The model under review builds one solid part; all positions refer to its coordinate system, in mm. A direction names the side the tool comes from. Round coordinates to 2 decimals unless told otherwise and drop trailing zeros. Write each loop counter-clockwise with the first axis right and the second up, starting at its lowest first coordinate (ties: lowest second). Pieces come first, ordered by that corner, then holes. Notation, with made-up numbers: (35, 84) - (79, 84) arc R33 cw to (79, 123) - close; hole circle Ø10 at (0, -24.75). An arc over 180 degrees is marked (long way). Use one line per item in the form item = value.
from build123d import *

# Parameters (mm, degrees)
FEMALE_HEX_STANDOFF_SKETCH_R  = 1.51
FEMALE_HEX_STANDOFF_DEPTH     = 5
STUD_ROOT_SKETCH_R            = 1.85
STUD_ROOT_DEPTH               = 0.45
MALE_THREAD_ENVELOPE_START    = -8
MALE_THREAD_ENVELOPE_SKETCH_R = 1.5
MALE_THREAD_ENVELOPE_DEPTH    = 8


with BuildPart() as part:
    # Female_hex_standoff_Sketch → Female_hex_standoff (new body)
    with BuildSketch(Plane.XY):
        Polygon((3.175426481, 0), (1.58771324, 2.75), (-1.58771324, 2.75), (-3.175426481, 0), (-1.58771324, -2.75), (1.58771324, -2.75), align=None)
        Circle(FEMALE_HEX_STANDOFF_SKETCH_R, mode=Mode.SUBTRACT)
    extrude(amount=FEMALE_HEX_STANDOFF_DEPTH)

    # Stud_root_Sketch → Stud_root (add)
    with BuildSketch(Plane.XY):
        Circle(STUD_ROOT_SKETCH_R)
    extrude(amount=STUD_ROOT_DEPTH)

    # Male_thread_envelope_Sketch → Male_thread_envelope (add)
    with BuildSketch(Plane.XY.offset(MALE_THREAD_ENVELOPE_START)):
        Circle(MALE_THREAD_ENVELOPE_SKETCH_R)
    extrude(amount=MALE_THREAD_ENVELOPE_DEPTH)


solid = part.part
(1) The part is to be moulded in two halves that separate along X. For faces 1 (the cylindrical face through (-1.5, 0.07, -4.06)), 2 (the cylindrical face through (-0.197, 1.497, 2.693)), 3 (the flat face through (0, 2.75, 2)), say which applies: +X half, -X half, draft (parallel to the pull), parting line (faces both ways), or undercut.
Geometry results:
face_1 = parting line
face_2 = undercut
face_3 = draft
(2) Add section A-A on x = 0. Write out the cut boundary in (y, z).
Geometry results:
outline = (-2.75, 0) - (-1.5, 0) - (-1.5, -8) - (1.5, -8) - (1.5, 0) - (2.75, 0) - (2.75, 5) - (1.51, 5) - (1.51, 0.45) - (-1.51, 0.45) - (-1.51, 5) - (-2.75, 5) - close
(3) Machinability: for faces 4 (the flat face through (1.4, 1.3, 0)), 5 (the flat face through (0, 0, 0.45)), 6 (the flat face through (2.37, -1.394, 2.465)), which of the approach directions +Z, -Z, +X, -X, +Y, -Y give a long, thin tool a straight path to every point of the face, cutting with its end or side? Answer none if there is none.
Geometry results:
face_4 = -Z
face_5 = +Z
face_6 = +Z, -Z, +X, -Y
(4) Insertion check: P1, Ø1.5, axis at x = 0, y = 0.5, coming from the +Z side. The pin has a flat end and moves straight along its axis. Give the tip position at first contact, or say it passes through.
Geometry results:
P1 = 0.45
(5) Add section C-C on z = -1.75. Write out the cut boundary in (x, y).
Geometry results:
outline = circle Ø3 at (0, 0)
(6) To check wall thickness, follow L1, parallel to Y at x = 0, z = 2.45; L2, parallel to Z at x = -0.5, y = -1.9; L3, parallel to Z at x = 0.25, y = 0.2. State the ranges of each line that lie inside material, in increasing order.
Geometry results:
L1 = -2.75 to -1.51, 1.51 to 2.75
L2 = 0 to 5
L3 = -8 to 0.45
(7) Add section D-D on y = -1.7. Write out the cut boundary in (x, z), then the cut area to 3 significant figures.
Geometry results:
outline = (-2.19, 0) - (2.19, 0) - (2.19, 5) - (-2.19, 5) - close
area = 21.9 mm2
(8) Add section B-B on y = 0.4. Write out the cut boundary in (x, z), then the cut area to 3 significant figures.
Geometry results:
outline = (-2.94, 0) - (-1.45, 0) - (-1.45, -8) - (1.45, -8) - (1.45, 0) - (2.94, 0) - (2.94, 5) - (1.46, 5) - (1.46, 0.45) - (-1.46, 0.45) - (-1.46, 5) - (-2.94, 5) - close
area = 39.3 mm2
